Here's how the part is built. I have some questions about the finished solid (model axes, mm). Face numbers are marked on the shaded views. A direction names the side the tool comes from. Round coordinates to 2 decimals unless told otherwise and drop trailing zeros. Write each loop counter-clockwise with the first axis right and the second up, starting at its lowest first coordinate (ties: lowest second). Pieces come first, ordered by that corner, then holes. Notation, with made-up numbers: M 38,75.5 L 54,75.5 A17 ccw 54,107.5 Z; hole C 69,37.25 d7. An arc over 180 degrees is marked long. Write item = value, one per line. Start each with the question number.
(1) I want a section at B-B (z = 4.25). List the corners of the cut face in (x, y) for me.
(2) Will this pin go through, and if not, where does the flat tip stop? pin 1 Ø1 at (x, z) = (-1, 4) entering from +Y.
(3) I need wall thicknesses on line 1 along X through (y, z) = (3.5, 4.5); line 2 along Y through (x, z) = (-4.5, 5.5). Which ranges of each line are inside material? Lowest first, please.
(4) I want a section at A-A (y = 7.25). List the corners of the cut face in (x, z) for me, and give its area (3 significant figures).
(5) I want a section at C-C (x = -5.5). List the corners of the cut face in (y, z) for me.
(6) If we mould it in two halves opening along Z, with no side actions, what happens to the marked faces 3, 4, 5 and 6? For each: released by +Z, released by -Z, zero draft, split by the parting line, or undercut.
(7) On a 3-axis mill with a long thin cutter (end or side, diameter ignored), from which of +Z, -Z, +X, -X, +Y, -Y can I reach the whole of each face in a straight line? I mean the marked faces 1 and 2. Say none if no direction works.
```python
from build123d import *

# Parameters (mm, degrees)
SKETCH5_W           = 15
SKETCH5_H           = 15
SKETCH5_W_2         = 13
SKETCH5_H_2         = 13
BOSS_EXTRUDE1_DEPTH = 10
SKETCH6_W           = 15
SKETCH6_H           = 1
BOSS_EXTRUDE2_DEPTH = 15


with BuildPart() as part:
    # Sketch5 → Boss-Extrude1 (new body)
    with BuildSketch(Plane(origin=(0, 0, 0), x_dir=(1, 0, 0), z_dir=(0, 1, 0))):
        Rectangle(SKETCH5_W, SKETCH5_H)
        Rectangle(SKETCH5_W_2, SKETCH5_H_2, mode=Mode.SUBTRACT)
    extrude(amount=BOSS_EXTRUDE1_DEPTH)

    # Sketch6 → Boss-Extrude2 (add)
    with BuildSketch(Plane(origin=(0, 0, -7.5), x_dir=(-1, 0, 0), z_dir=(0, 0, -1))):
        with Locations((0, -0.5)):
            Rectangle(SKETCH6_W, SKETCH6_H)
    extrude(amount=-BOSS_EXTRUDE2_DEPTH)


solid = part.part
```
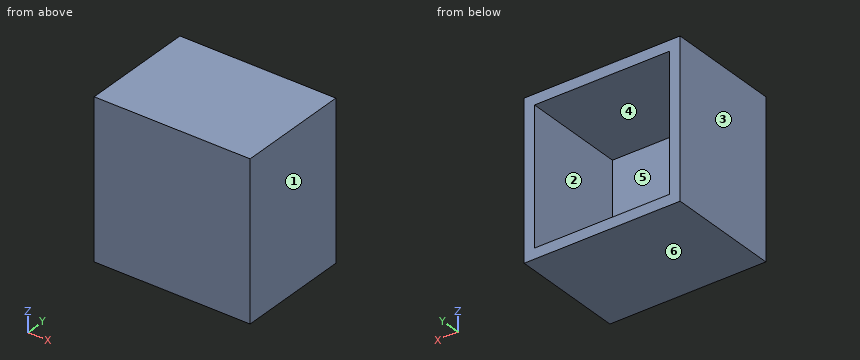
Returned:
q1.outline = M -7.5,-1 L 7.5,-1 L 7.5,10 L 6.5,10 L 6.5,0 L -6.5,0 L -6.5,10 L -7.5,10 Z
q2.pin_1 = 0
q3.line_1 = -7.5 to -6.5, 6.5 to 7.5
q3.line_2 = -1 to 0
q4.outline = M -7.5,-7.5 L 7.5,-7.5 L 7.5,7.5 L -7.5,7.5 Z; hole M -6.5,-6.5 L 6.5,-6.5 L 6.5,6.5 L -6.5,6.5 Z
q4.area = 56.0 mm²
q5.outline = M -1,-7.5 L 10,-7.5 L 10,-6.5 L 0,-6.5 L 0,6.5 L 10,6.5 L 10,7.5 L -1,7.5 Z
q6.face_3 = zero draft
q6.face_4 = undercut
q6.face_5 = undercut
q6.face_6 = released by -Z
q7.face_1 = +Z, -Z, +X, +Y, -Y
q7.face_2 = +Y
